Here's how the part is built. I have some questions about the finished solid (model axes, mm). A direction names the side the tool comes from. Coordinates: 2 decimals unless noted, no trailing zeros. Write each loop counter-clockwise with the first axis right and the second up, starting at its lowest first coordinate (ties: lowest second). Pieces come first, ordered by that corner, then holes. Notation, with made-up numbers: (-28.75, 51) -> (-17.75, 51) arc R6 ccw to (-17.75, 56) -> close; hole circle Ø10 at (-31.75, 26.5). An arc over 180 degrees is marked (long way). Answer in a Markdown table with one row per item. Add a question column.
from build123d import *

# Parameters (mm, degrees)
CORTAR_REVOLUCI_N1_START = 13.6
CORTAR_REVOLUCI_N1_DEPTH = 6
MATRIZC1_COUNT           = 3
CROQUIS4_R               = 0.75
CORTAR_EXTRUIR1_DEPTH    = 28.824090282


# Read off the part's stored shape, not the designer's step: Cortar-Revolución1
with BuildPart() as part:
    # Croquis1 → Revolución1 (revolve)
    with BuildSketch(Plane.YZ):
        with BuildLine():
            Line((-3, 0), (-3, 10))
            ThreePointArc((-3, 10), (-7.036805787, 13.954628111), (-7.291090453, 19.6))
            Line((-7.291090453, 19.6), (-4.445222154, 19.6))
            ThreePointArc((-4.445222154, 19.6), (-4.295338521, 19.444092675), (-4.45702764, 19.300465287))
            ThreePointArc((-4.45702764, 19.300465287), (-4.57485069, 19.273071665), (-4.655330258, 19.182762635))
            ThreePointArc((-4.655330258, 19.182762635), (-4.279724841, 14.326202011), (0, 12))
            Line((0, 12), (0, 0))
            Line((0, 0), (0, -6))
            Line((0, -6), (-1, -6))
            Line((-1, -6), (-1, 0))
            Line((-1, 0), (-3, 0))
        make_face()
    revolve(axis=Axis((0, 0, 0), (0, 0, -1)))

    # Cortar-Revolución1 outline → Cortar-Revolución1 (cut)
    with BuildSketch(Plane.XY.offset(CORTAR_REVOLUCI_N1_START)):
        Polygon((0.945938118, -9), (0.805683263, -7.665564198), (0.387742836, -3.689126657), (0.21020847, -2), (-0.21020847, -2), (-0.387742836, -3.689126657), (-0.805683263, -7.665564198), (-0.945938118, -9), align=None)
    cortar_revoluci_n1 = extrude(amount=CORTAR_REVOLUCI_N1_DEPTH, mode=Mode.SUBTRACT)

    # MatrizC1: Cortar-Revolución1 ×3 about axis
    matrizc1_axis = Axis((0, 0, 0), (0, 0, 1))
    for i in range(1, MATRIZC1_COUNT):
        add(cortar_revoluci_n1.rotate(matrizc1_axis, i * 360 / MATRIZC1_COUNT), mode=Mode.SUBTRACT)

    # Croquis4 → Cortar-Extruir1 (cut, through all)
    with BuildSketch(Plane.XY.offset(19.6)):
        Circle(CROQUIS4_R)
    extrude(amount=-CORTAR_EXTRUIR1_DEPTH, mode=Mode.SUBTRACT)


solid = part.part
Q1. Imagine slicing it at C-C on z = 7.75. Please give me the cut outline in (x, y), plus the area to 3 significant figures.
Q2. If we mould it in two halves opening along Y, with no side actions, what happens to faces 1 (the flat face through (5.595, 2.491, 16.558)), 2 (the flat face through (-0.64, -6.09, 16.56)), 3 (the cylindrical face through (0, 3, 5))? For each: pulls with the +Y half, pulls with the -Y half, needs draft (parallel to the pull), parting line crosses it, or undercut.
Q3. Imagine slicing it at A-A on y = 0. Please give me the cut outline in (x, z), plus the area to 3 significant figures.
Q4. Imagine slicing it at D-D on y = -6.5. Please give me the cut outline in (x, z).
Q5. Imagine slicing it at B-B on x = 0. Please give me the cut outline in (y, z), plus the area to 3 significant figures.
Q6. I'm going to push flat-ended pins straight in: P1, Ø5, axis at x = -3.5, y = -5, coming from the -Z side; P2, Ø6, axis at y = -5.5, z = 4.5, coming from the +X side; P3, Ø5, axis at x = 4.5, z = 3.5, coming from the -Y side. Where does each tip first touch, or does it pass through?
Q7. I need wall thicknesses on line 1 (Y direction, x = 0, z = -1); line 2 (X direction, y = 0, z = 3.75). Which ranges of each line are inside material? Lowest first, please. Write a range as [from, to].
Q8. For faces 4 (the cylindrical face through (-0.75, 0.03, 3.15)), 5 (the cylindrical face through (1, 0, -3)), 6 (the flat face through (0.646, -6.147, 16.558)), 7 (the flat face through (-5, -3, 19.6)), 8 (the flat face through (-5.647, 2.514, 16.558)), which set-ups out of +Z, -Z, +X, -X, +Y, -Y let a thin tool reach every point of the face, with its end or its side?
Result sheet:
| question | item | result |
|---|---|---|
| 1 | outline | circle Ø6 at (0, 0); hole circle Ø1.5 at (0, 0) |
| 1 | area | 26.5 mm^2 |
| 2 | face 1 | undercut |
| 2 | face 2 | pulls with the -Y half |
| 2 | face 3 | parting line crosses it |
| 3 | outline | (-7.29, 19.6) arc R7.71 ccw to (-3, 10) -> (-3, 0) -> (-1, 0) -> (-1, -6) -> (-0.75, -6) -> (-0.75, 12.06) arc R5.1 cw to (-4.66, 19.18) arc R0.2 cw to (-4.46, 19.3) arc R0.15 ccw (long way) to (-4.45, 19.6) -> close; (0.75, -6) -> (1, -6) -> (1, 0) -> (3, 0) -> (3, 10) arc R7.71 ccw to (7.29, 19.6) -> (4.45, 19.6) arc R0.15 ccw (long way) to (4.46, 19.3) arc R0.2 cw to (4.66, 19.18) arc R5.1 cw to (0.75, 12.06) -> close |
| 3 | area | 109 mm^2 |
| 4 | outline | (-3.3, 19.6) arc R4.14 ccw (long way) to (3.3, 19.6) -> (0.68, 19.6) -> (0.68, 13.6) -> (-0.68, 13.6) -> (-0.68, 19.6) -> close |
| 5 | outline | (-6.87, 13.6) arc R7.71 ccw to (-3, 10) -> (-3, 0) -> (-1, 0) -> (-1, -6) -> (-0.75, -6) -> (-0.75, 12.06) arc R5.1 cw to (-3.71, 13.6) -> close; (0.75, -6) -> (1, -6) -> (1, 0) -> (3, 0) -> (3, 10) arc R7.71 ccw to (7.29, 19.6) -> (4.45, 19.6) arc R0.15 ccw (long way) to (4.46, 19.3) arc R0.2 cw to (4.66, 19.18) arc R5.1 cw to (0.75, 12.06) -> close |
| 5 | area | 92.1 mm^2 |
| 6 | P1 | stops at z = 10.29 |
| 6 | P2 | stops at x = 1.66 |
| 6 | P3 | stops at y = -2.24 |
| 7 | line 1 | y = [-1, -0.75], [0.75, 1] |
| 7 | line 2 | x = [-3, -0.75], [0.75, 3] |
| 8 | face 4 | +Z, -Z |
| 8 | face 5 | -Z |
| 8 | face 6 | +Z, -Y |
| 8 | face 7 | +Z, +X, -X, +Y, -Y |
| 8 | face 8 | +Z |
